Design review of the part shown in the three views and the two pictorial views. Dimensions are in mm from the part's minimum x, y and z. A direction names the side the tool comes from. Round coordinates to 2 decimals unless told otherwise and drop trailing zeros. Order: outer loops, then holes, each group sorted by start corner. A loop starts at its lowest first (then second) coordinate and runs counter-clockwise, first axis right, second up.
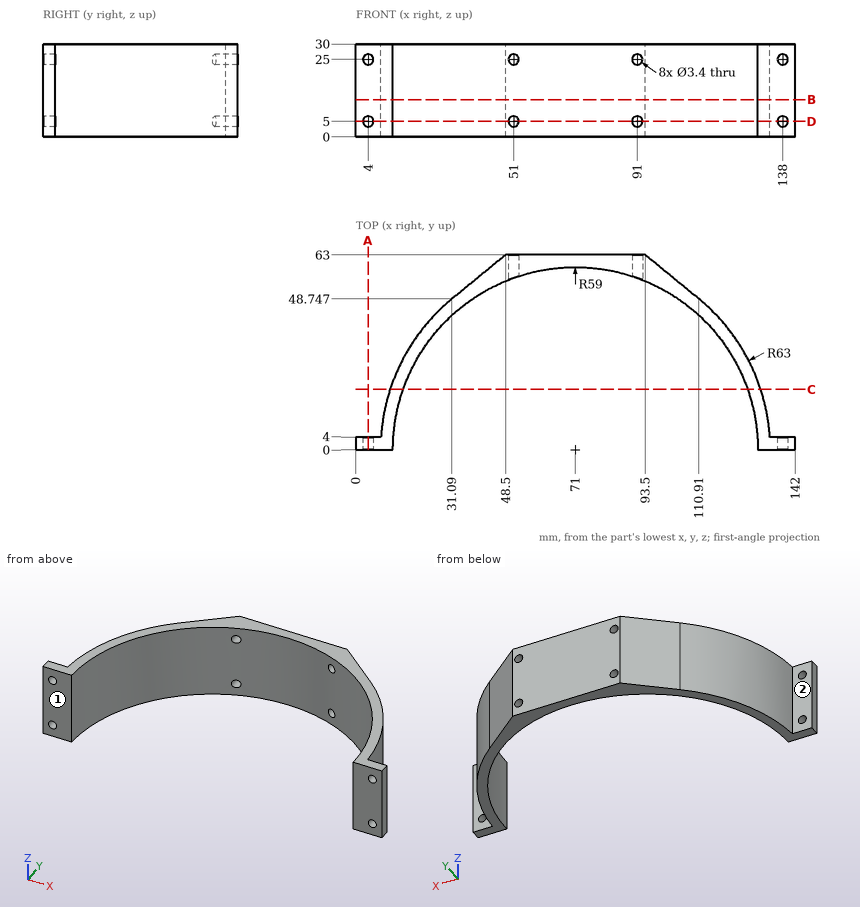
(1) Insertion check: pin 1 (6 mm diameter, centred on x = 36.5, z = 10, fed in from +Y); pin 2 (3 mm diameter, centred on y = 23, z = 11.5, fed in from +X); pin 3 (1.5 mm diameter, centred on x = 36, z = 12, fed in from +Y); pin 4 (4.5 mm diameter, centred on x = 138, z = 25, fed in from -Y). Each pin has a flat end and moves straight along its axis. Give the tip position at first contact, or say it passes through.
Data:
pin 1: stops at y = 55.63
pin 2: stops at x = 130.22
pin 3: stops at y = 53.38
pin 4: stops at y = 0
(2) To check wall thickness, follow probe 1 along Z at (x, y) = (4, 2.35); probe 2 along X at (y, z) = (36, 11.5) (1 decimal); probe 3 along Y at (x, z) = (136, 7.5). State the ranges of each line that lie inside material, in increasing order.
Data:
probe 1: z = 0 to 3.3, 6.7 to 23.3, 26.7 to 30
probe 2: x = 19.3 to 24.3, 117.7 to 122.7
probe 3: y = 0 to 4
(3) Consider section C-C (y = 19.5). Write out the cut boundary in (x, z) (1 decimal), and give its area (3 significant figures).
Data:
outline: (11.1, 0) - (15.3, 0) - (15.3, 30) - (11.1, 30) - close; (126.7, 0) - (130.9, 0) - (130.9, 30) - (126.7, 30) - close
area: 253 mm2
(4) For the marked faces 1 and 2, list the 3-axis set-ups (+Z, -Z, +X, -X, +Y, -Y) from which the entire face can be reached by the end or side of a thin tool; tool diameter is ignored.
Data:
face 1: +Z, -Z, +X, -X, -Y
face 2: +Z, -Z, -X, +Y
(5) Consider section D-D (z = 5). Write out the cut boundary in (x, y) (1 decimal).
Data:
outline: (0, 0) - (2.3, 0) - (2.3, 4) - (0, 4) - close; (5.7, 0) - (12, 0) arc R59 cw to (49.3, 54.9) - (49.3, 63) - (48.5, 63) - (31.1, 48.7) arc R63 ccw to (8.1, 4) - (5.7, 4) - close; (52.7, 56.1) arc R59 cw to (89.3, 56.1) - (89.3, 63) - (52.7, 63) - close; (92.7, 54.9) arc R59 cw to (130, 0) - (136.3, 0) - (136.3, 4) - (133.9, 4) arc R63 ccw to (110.9, 48.7) - (93.5, 63) - (92.7, 63) - close; (139.7, 0) - (142, 0) - (142, 4) - (139.7, 4) - close
(6) Consider section B-B (z = 12). Write out the cut boundary in (x, y).
Data:
outline: (0, 0) - (12, 0) arc R59 cw to (130, 0) - (142, 0) - (142, 4) - (133.87, 4) arc R63 ccw to (110.91, 48.75) - (93.5, 63) - (48.5, 63) - (31.09, 48.75) arc R63 ccw to (8.13, 4) - (0, 4) - close
(7) Consider section A-A (x = 4). Write out the cut boundary in (y, z).
Data:
outline: (0, 0) - (4, 0) - (4, 3.3) - (0, 3.3) - close; (0, 6.7) - (4, 6.7) - (4, 23.3) - (0, 23.3) - close; (0, 26.7) - (4, 26.7) - (4, 30) - (0, 30) - close
